Verification items for the finished model (mm, model axes). A direction names the side the tool comes from. Coordinates: 2 decimals unless noted, no trailing zeros. Write each loop counter-clockwise with the first axis right and the second up, starting at its lowest first coordinate (ties: lowest second). Pieces come first, ordered by that corner, then holes. Notation, with made-up numbers: (58, 28) -> (63, 28) arc R30 cw to (63, 56) -> close; hole circle Ø6 at (31.25, -24). An arc over 180 degrees is marked (long way). Write item = value, one per line. Start each with the question number.
(1) Section check B-B (x = 22). Record the cut outline in (y, z), plus the area to 3 significant figures.
(2) Mould release check, pull along Z, two halves, no side actions. Record for faces 1 (the face through (-29, 8.4, 0)), 2 (the face through (29, 24, 24)): released by +Z, released by -Z, zero draft, split by the parting line, or undercut.
(3) Gauge pin test, flat ends, axial feed: pin 1 Ø5 at (y, z) = (6, 11) entering from +X; pin 2 Ø2.5 at (x, z) = (28.5, -24.5) entering from -Y; pin 3 Ø0.9 at (x, z) = (-28.5, -24.5) entering from -Y. Record the tip position at first contact, or that the pin passes through.
(4) Set-up check for faces 3 (the face through (27, 18.4, -25)), 4 (the face through (29, 5, 25)), 5 (the face through (-29, 24, -25)): record each of +Z, -Z, +X, -X, +Y, -Y from which the full face is reachable in a straight line by a thin tool's end or side.
(5) Section check A-A (z = 9.5). Record the cut outline in (x, y), plus the area to 3 significant figures.
(6) Material ranges on probe 1 along X at (y, z) = (1.6, 24.5); probe 2 along X at (y, z) = (8.75, 7); probe 3 along Z at (x, y) = (26, 17.5), recorded low to high. Write a range as [from, to].
```python
from build123d import *

# Parameters (mm, degrees)
SKETCH_1_R          = 3
EXTRUDE_1_DEPTH     = 18.4
EXTRUDE_1_2_DEPTH   = 18.4
EXTRUDE_1_3_DEPTH   = 18.4
EXTRUDE_1_4_DEPTH   = 18.4
SKETCH_2_R          = 1.45
CUT_EXTRUDE_1_DEPTH = 5
SKETCH_3_R          = 5
EXTRUDE_2_DEPTH     = 3
EXTRUDE_START       = -7
EXTRUDE_3_DEPTH     = 3
CHAMFER_1_SIZE      = 0.5
SKETCH_5_R          = 1.9
EXTRUDE_4_DEPTH     = 5.6
CHAMFER_2_SIZE      = 0.5
CHAMFER_3_SIZE      = 2
FILLET_1_R          = 1


with BuildPart() as part:
    # Sketch 1 → Extrude 1 (new body)
    with BuildSketch(Plane(origin=(0, 0, 0), x_dir=(1, 0, 0), z_dir=(0, 1, 0))):
        with Locations(Location((-29, 24.5, 0), (0, 0, 270))):
            Circle(SKETCH_1_R)
    extrude(amount=EXTRUDE_1_DEPTH)


with BuildPart() as body_2:
    # Sketch 1 → Extrude 1 2 (new body)
    with BuildSketch(Plane(origin=(0, 0, 0), x_dir=(1, 0, 0), z_dir=(0, 1, 0))):
        with Locations(Location((29, 24.5, 0), (0, 0, 90))):
            Circle(SKETCH_1_R)
    extrude(amount=EXTRUDE_1_2_DEPTH)


with BuildPart() as body_3:
    # Sketch 1 → Extrude 1 3 (new body)
    with BuildSketch(Plane(origin=(0, 0, 0), x_dir=(1, 0, 0), z_dir=(0, 1, 0))):
        with Locations(Location((-29, -24.5, 0), (0, 0, 90))):
            Circle(SKETCH_1_R)
    extrude(amount=EXTRUDE_1_3_DEPTH)


with BuildPart() as body_4:
    # Sketch 1 → Extrude 1 4 (new body)
    with BuildSketch(Plane(origin=(0, 0, 0), x_dir=(1, 0, 0), z_dir=(0, 1, 0))):
        with Locations(Location((29, -24.5, 0), (0, 0, 270))):
            Circle(SKETCH_1_R)
    extrude(amount=EXTRUDE_1_4_DEPTH)


with BuildPart() as cut_extrude_1_tool:
    # Sketch 2 → Cut-Extrude 1 (new body)
    with BuildSketch(Plane.XZ):
        with Locations(Location((-29, 24.5, 0), (0, 0, 270))):
            Circle(SKETCH_2_R)
        with Locations(Location((29, 24.5, 0), (0, 0, 270))):
            Circle(SKETCH_2_R)
        with Locations(Location((-29, -24.5, 0), (0, 0, 270))):
            Circle(SKETCH_2_R)
        with Locations(Location((29, -24.5, 0), (0, 0, 270))):
            Circle(SKETCH_2_R)
    extrude(amount=-CUT_EXTRUDE_1_DEPTH)


with BuildPart() as part_1:
    add(part.part)

    # Cut-Extrude 1: cut by cut_extrude_1_tool
    add(cut_extrude_1_tool.part, mode=Mode.SUBTRACT)



with BuildPart() as body_2_1:
    add(body_2.part)

    # Cut-Extrude 1: cut by cut_extrude_1_tool
    add(cut_extrude_1_tool.part, mode=Mode.SUBTRACT)


with BuildPart() as body_3_1:
    add(body_3.part)

    # Cut-Extrude 1: cut by cut_extrude_1_tool
    add(cut_extrude_1_tool.part, mode=Mode.SUBTRACT)


with BuildPart() as body_4_1:
    add(body_4.part)

    # Cut-Extrude 1: cut by cut_extrude_1_tool
    add(cut_extrude_1_tool.part, mode=Mode.SUBTRACT)


with BuildPart() as part_2:
    add(part_1.part)

    add(body_2_1.part)  # Extrude 2 merges body 2

    add(body_3_1.part)  # Extrude 2 merges body 3

    add(body_4_1.part)  # Extrude 2 merges body 4
    # Sketch 3 → Extrude 2 (add)
    with BuildSketch(Plane(origin=(0, 18.4, 0), x_dir=(1, 0, 0), z_dir=(0, 1, 0))):
        with Locations(Location((29, 24.5, 0), (0, 0, 270))):
            Circle(SKETCH_3_R)
        with Locations(Location((29, -24.5, 0), (0, 0, 270))):
            Circle(SKETCH_3_R)
        with Locations(Location((-29, -24.5, 0), (0, 0, 270))):
            Circle(SKETCH_3_R)
        with Locations(Location((-29, 24.5, 0), (0, 0, 270))):
            Circle(SKETCH_3_R)
    extrude(amount=-EXTRUDE_2_DEPTH)

    # Sketch 4 → Extrude 3 (add)
    with BuildSketch(Plane(origin=(0, 18.4, 0), x_dir=(1, 0, 0), z_dir=(0, 1, 0)).offset(EXTRUDE_START)):
        Polygon((27.5, 23), (27.5, -23), (27.5, -26), (30.5, -26), (30.5, 26), (-30.5, 26), (-30.5, -26), (-27.5, -26), (-27.5, -23), (-27.5, 23), align=None)
    extrude(amount=-EXTRUDE_3_DEPTH)

    # Chamfer 1
    chamfer_1_edges = [part_2.edges().sort_by_distance(p)[0] for p in [
        (-29, 0, -23.05),
        (-29, 0, -27.5),
        (29, 0, -21.5),
        (29, 0, -23.05),
        (-29, 0, 27.5),
        (-29, 0, 25.95),
        (29, 0, 21.5),
        (29, 0, 25.95),
    ]]
    chamfer(chamfer_1_edges, length=CHAMFER_1_SIZE)

    # Sketch 5 → Extrude 4 (add)
    with BuildSketch(Plane(origin=(0, 18.4, 0), x_dir=(1, 0, 0), z_dir=(0, 1, 0))):
        with Locations(Location((29, 24.5, 0), (0, 0, 270))):
            Circle(SKETCH_5_R)
        with Locations(Location((29, -24.5, 0), (0, 0, 270))):
            Circle(SKETCH_5_R)
        with Locations(Location((-29, -24.5, 0), (0, 0, 270))):
            Circle(SKETCH_5_R)
        with Locations(Location((-29, 24.5, 0), (0, 0, 270))):
            Circle(SKETCH_5_R)
    extrude(amount=EXTRUDE_4_DEPTH)

    # Chamfer 2
    chamfer_2_edges = [part_2.edges().sort_by_distance(p)[0] for p in [
        (29, 24, -26.4),
        (29, 24, 22.6),
        (-29, 24, 22.6),
        (-29, 24, -26.4),
    ]]
    chamfer(chamfer_2_edges, length=CHAMFER_2_SIZE)

    # Chamfer 3
    chamfer_3_edges = [part_2.edges().sort_by_distance(p)[0] for p in [
        (-29, 15.4, -27.5),
        (-29, 18.4, -29.5),
        (29, 15.4, -21.5),
        (29, 18.4, -29.5),
        (-29, 15.4, 27.5),
        (-29, 18.4, 19.5),
        (29, 15.4, 21.5),
        (29, 18.4, 19.5),
    ]]
    chamfer(chamfer_3_edges, length=CHAMFER_3_SIZE - 0.0001)  # a hair under: the kernel refuses the full size

    # Fillet 1
    fillet_1_edges = [part_2.edges().sort_by_distance(p)[0] for p in [
        (-30.5, 9.9, -21.901923789),
        (-27.5, 9.9, -21.901923789),
        (-26.401923789, 9.9, -26),
        (-26.401923789, 9.9, -23),
        (27.5, 9.9, -21.901923789),
        (26.401923789, 9.9, -26),
        (26.401923789, 9.9, -23),
        (30.5, 9.9, -21.901923789),
        (-27.5, 9.9, 21.901923789),
        (-30.5, 9.9, 21.901923789),
        (30.5, 9.9, 21.901923789),
        (27.5, 9.9, 21.901923789),
    ]]
    fillet(fillet_1_edges, radius=FILLET_1_R)


solid = part_2.part
```
Response:
q1.outline = (8.4, -26) -> (11.4, -26) -> (11.4, -23) -> (8.4, -23) -> close
q1.area = 9.00 mm2
q2.face_1 = undercut
q2.face_2 = zero draft
q3.pin_1 = 30.5
q3.pin_2 = 0.2
q3.pin_3 = 5
q4.face_3 = +Y
q4.face_4 = -Y
q4.face_5 = +Z, -Z, +X, -X, +Y
q5.outline = (-30.5, 8.4) -> (-27.5, 8.4) -> (-27.5, 11.4) -> (-30.5, 11.4) -> close; (27.5, 8.4) -> (30.5, 8.4) -> (30.5, 11.4) -> (27.5, 11.4) -> close
q5.area = 18.0 mm2
q6.probe_1 = [-32, -30.45], [-27.55, -26], [26, 27.55], [30.45, 32]
q6.probe_2 = [-30.5, -27.5], [27.5, 30.5]
q6.probe_3 = [-26.99, -22.01], [22.01, 26.99]
